For this review, take the finished solid that the model builds, in its own axes (mm). Face numbers are marked on the shaded views. A direction names the side the tool comes from. Round coordinates to 2 decimals unless told otherwise and drop trailing zeros. Order: outer loops, then holes, each group sorted by start corner. A loop starts at its lowest first (then second) coordinate and runs counter-clockwise, first axis right, second up. Notation, with made-up numbers: M 8,31.5 L 30,31.5 A26 ccw 30,52.5 Z; hole C 0.25,-19.75 d8. An arc over 180 degrees is marked long. Write item = value, one per line. Start each with the question number.
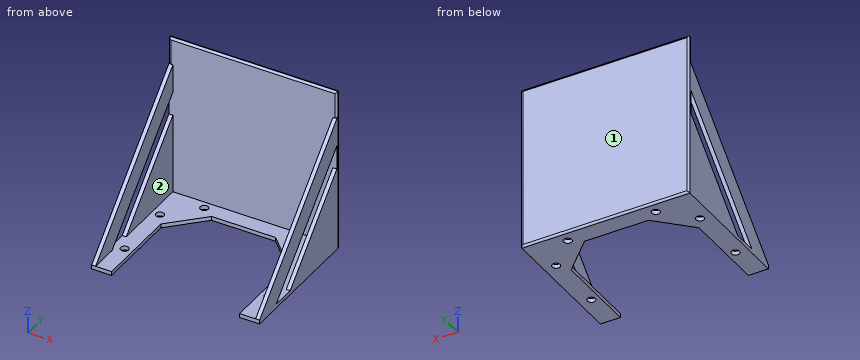
from build123d import *

# Parameters (mm, degrees)
BOSS_EXTRUDE1_DEPTH = 3.175
SKETCH3_R           = 3.175
CUT_EXTRUDE1_DEPTH  = 86.976283948
SKETCH4_W           = 133.35
SKETCH4_H           = 3.175
BOSS_EXTRUDE2_DEPTH = 127
BOSS_EXTRUDE3_DEPTH = 3.175
BOSS_EXTRUDE4_DEPTH = 3.175
FILLET2_R           = 1.5875


with BuildPart() as part:
    # Sketch2 → Boss-Extrude1 (new body)
    with BuildSketch(Plane.XY):
        Polygon((-50.8, -54.187499956), (-50.8, 12.912499956), (-25.4, 38.312499956), (25.4, 38.312499956), (50.8, 12.912499956), (50.8, -54.187499956), (66.675, -54.187499956), (66.675, 54.187499956), (-66.675, 54.187499956), (-66.675, -54.187499956), align=None)
    extrude(amount=BOSS_EXTRUDE1_DEPTH)

    # Sketch3 → Cut-Extrude1 (cut, through all)
    with BuildSketch(Plane.XY.offset(3.175)):
        with Locations((-57.15, -25.612499956)):
            Circle(SKETCH3_R)
        with Locations((-57.15, 22.437499956)):
            Circle(SKETCH3_R)
        with Locations((-34.925, 44.662499956)):
            Circle(SKETCH3_R)
        with Locations(Location((34.925, 44.662499956, 0), (0, 0, 180))):
            Circle(SKETCH3_R)
        with Locations(Location((57.15, 22.437499956, 0), (0, 0, 180))):
            Circle(SKETCH3_R)
        with Locations(Location((57.15, -25.612499956, 0), (0, 0, 180))):
            Circle(SKETCH3_R)
    extrude(amount=-CUT_EXTRUDE1_DEPTH, mode=Mode.SUBTRACT)

    # Sketch4 → Boss-Extrude2 (add)
    with BuildSketch(Plane.XY.offset(3.175)):
        with Locations((0, 52.599999956)):
            Rectangle(SKETCH4_W, SKETCH4_H)
    extrude(amount=BOSS_EXTRUDE2_DEPTH)

    # Sketch5 → Boss-Extrude3 (add)
    with BuildSketch(Plane.ZY.offset(66.675)):
        Polygon((3.175, -12.487500044), (66.675, 51.012499956), (3.175, 51.012499956), align=None)
        Polygon((108.374999912, 51.012499956), (3.175, -54.187499956), (3.175, -31.736859653), (85.924359609, 51.012499956), align=None)
    extrude(amount=-BOSS_EXTRUDE3_DEPTH)

    # Sketch6 → Boss-Extrude4 (add)
    with BuildSketch(Plane(origin=(66.675, 0, 0), x_dir=(0, 0, -1), z_dir=(1, 0, 0))):
        Polygon((-108.374999912, 51.012499956), (-3.175, -54.187499956), (-3.175, -31.736859653), (-85.924359609, 51.012499956), align=None)
        Polygon((-3.175, -12.487500044), (-66.675, 51.012499956), (-3.175, 51.012499956), align=None)
    extrude(amount=-BOSS_EXTRUDE4_DEPTH)

    # Fillet2
    fillet2_edges = [part.edges().sort_by_distance(p)[0] for p in [
        (66.675, 54.187499956, 65.0875),
        (0, 54.187499956, 130.175),
        (-66.675, 54.187499956, 65.0875),
        (0, 54.187499956, 0),
        (66.675, 51.012499956, 119.274999956),
        (0, 51.012499956, 130.175),
        (-66.675, 51.012499956, 119.274999956),
    ]]
    fillet(fillet2_edges, radius=FILLET2_R - 0.0001)  # a hair under: the kernel refuses the full size


solid = part.part
(1) For line 1 along X through (y, z) = (14, 11) (3 decimals); line 2 along Y through (x, z) = (57, 1); line 3 along Y through (x, z) = (-0.5, 66), list the stretches that pass through material, from the lowest coordinate up.
(2) For the marked faces 1 and 2, list the 3-axis set-ups (+Z, -Z, +X, -X, +Y, -Y) from which the entire face can be reached by the end or side of a thin tool; tool diameter is ignored.
(3) We need section C-C, the plane y = -46. Write out the cut boundary in (x, z) (1 decimal), then the cut area to 3 significant figures.
(4) Insertion check: pin 1 (4 mm diameter, centred on x = -57.15, y = 22.44, fed in from -Z); pin 2 (2.5 mm diameter, centred on x = -1.5, z = 2, fed in from -Y); pin 3 (8 mm diameter, centred on x = -45.5, y = 39, fed in from -Z); pin 4 (1.5 mm diameter, centred on x = -51, y = 42.5, fed in from +Z) (3 decimals). Each pin has a flat end and moves straight along its axis. Give the tip position at first contact, or say it passes through.
(5) We need section B-B, the plane z = 12. Write out the cut boundary in (x, y) (1 decimal), then the cut area to 3 significant figures.
(6) We need section A-A, the plane x = -57.15. State how many separate pieces and enclosed holes the cut face has, then the cut area to 3 significant figures.
Values:
q1.line_1 = -66.675 to -63.5, 63.5 to 66.675
q1.line_2 = -54.19 to -28.78, -22.44 to 19.27, 25.61 to 54.07
q1.line_3 = 51.01 to 54.19
q2.face_1 = +Z, -Z, +X, -X, +Y
q2.face_2 = +Z, -Y
q3.outline = M -66.7,0 L -50.8,0 L -50.8,3.2 L -63.5,3.2 L -63.5,11.4 L -66.7,11.4 Z; M 50.8,0 L 66.7,0 L 66.7,11.4 L 63.5,11.4 L 63.5,3.2 L 50.8,3.2 Z
q3.area = 153 mm²
q4.pin_1 = through
q4.pin_2 = 38.31
q4.pin_3 = 0
q4.pin_4 = 3.175
q5.outline = M -66.7,-45.4 L -63.5,-45.4 L -63.5,-22.9 L -66.7,-22.9 Z; M -66.7,-3.7 L -63.5,-3.7 L -63.5,51 L 63.5,51 L 63.5,-3.7 L 66.7,-3.7 L 66.7,52.6 A1.6 ccw 65.1,54.2 L -65.1,54.2 A1.6 ccw -66.7,52.6 Z; M 63.5,-45.4 L 66.7,-45.4 L 66.7,-22.9 L 63.5,-22.9 Z
q5.area = 912 mm²
q6.separate_pieces = 3
q6.enclosed_holes = 0
q6.area = 705 mm²
